```python
from build123d import *

# Parameters (mm, degrees)
BOSS_EXTRU_1_DEPTH = 812.8


with BuildPart() as part:
    # Esquisse1 → Boss.-Extru.1 (new body)
    with BuildSketch(Plane.XY.offset(406.4)):
        with BuildLine():
            Line((25.4, -22.86), (25.4, 22.86))
            ThreePointArc((25.4, 22.86), (24.656051224, 24.656051224), (22.86, 25.4))
            Line((22.86, 25.4), (-22.86, 25.4))
            ThreePointArc((-22.86, 25.4), (-24.656051224, 24.656051224), (-25.4, 22.86))
            Line((-25.4, 22.86), (-25.4, -22.86))
            ThreePointArc((-25.4, -22.86), (-24.656051224, -24.656051224), (-22.86, -25.4))
            Line((-22.86, -25.4), (22.86, -25.4))
            ThreePointArc((22.86, -25.4), (24.656051224, -24.656051224), (25.4, -22.86))
        make_face()
        with BuildLine():
            Line((-20.1168, 22.352), (20.1168, 22.352))
            ThreePointArc((20.1168, 22.352), (21.697325077, 21.697325077), (22.352, 20.1168))
            Line((22.352, 20.1168), (22.352, -20.1168))
            ThreePointArc((22.352, -20.1168), (21.697325077, -21.697325077), (20.1168, -22.352))
            Line((20.1168, -22.352), (-20.1168, -22.352))
            ThreePointArc((-20.1168, -22.352), (-21.697325077, -21.697325077), (-22.352, -20.1168))
            Line((-22.352, -20.1168), (-22.352, 20.1168))
            ThreePointArc((-22.352, 20.1168), (-21.697325077, 21.697325077), (-20.1168, 22.352))
        make_face(mode=Mode.SUBTRACT)
    extrude(amount=-BOSS_EXTRU_1_DEPTH)


solid = part.part
```
Source: CAD feature listing. Evaluate the final solid. Frame: model axes, mm. A direction names the side the tool comes from. Give positions to 0.01 mm unless a question says otherwise; leave off trailing zeros. Write each loop counter-clockwise with the first axis right and the second up, starting at its lowest first coordinate (ties: lowest second). Pieces come first, ordered by that corner, then holes. Notation, with made-up numbers: (-5, -31) - (45, -31) arc R21 cw to (45, -22) - close; hole circle Ø1 at (44, 88.25). An arc over 180 degrees is marked (long way). One line per item, written item: value. Start each with the question number.
Q1. Set-up query: faces 5 (the face through (-25.4, 0, 6)), 6 (the face through (0, -22.352, 6)). Return all of +Z, -Z, +X, -X, +Y, -Y with unobstructed straight access to the full face (end or side cutting, diameter ignored); none if empty.
Q2. Draft query along Y for faces 1 (the face through (0, 25.4, 6)), 2 (the face through (-23, 0, -406.4)), 3 (the face through (0, 22.352, 6)), 4 (the face through (0, -25.4, 6)). Return one class per face: +Y half, -Y half, draft (parallel to the pull), parting line (faces both ways), or undercut.
Q3. Material intervals for probe 1 along X at (y, z) = (17, 46.5); probe 2 along X at (y, z) = (20.5, 315.5), sorted ascending. Write a range as from..to.
Q4. Section query C-C, the plane z = 113.5. Return the cut outline in (x, y).
Q5. Section query A-A, the plane y = 12. Return the cut outline in (x, z).
Answer:
1. face 5: +Z, -Z, -X, +Y, -Y
1. face 6: +Z, -Z
2. face 1: +Y half
2. face 2: draft
2. face 3: undercut
2. face 4: -Y half
3. probe 1: x = -25.4..-22.35, 22.35..25.4
3. probe 2: x = -25.4..-22.32, 22.32..25.4
4. outline: (-25.4, -22.86) arc R2.54 ccw to (-22.86, -25.4) - (22.86, -25.4) arc R2.54 ccw to (25.4, -22.86) - (25.4, 22.86) arc R2.54 ccw to (22.86, 25.4) - (-22.86, 25.4) arc R2.54 ccw to (-25.4, 22.86) - close; hole (-22.35, -20.12) arc R2.24 ccw to (-20.12, -22.35) - (20.12, -22.35) arc R2.24 ccw to (22.35, -20.12) - (22.35, 20.12) arc R2.24 ccw to (20.12, 22.35) - (-20.12, 22.35) arc R2.24 ccw to (-22.35, 20.12) - close
5. outline: (-25.4, -406.4) - (-22.35, -406.4) - (-22.35, 406.4) - (-25.4, 406.4) - close; (22.35, -406.4) - (25.4, -406.4) - (25.4, 406.4) - (22.35, 406.4) - close
